The listing builds one solid part. Answer for the finished solid, in the listing's coordinates (mm). A direction names the side the tool comes from. Coordinates: 2 decimals unless noted, no trailing zeros. Write each loop counter-clockwise with the first axis right and the second up, starting at its lowest first coordinate (ties: lowest second). Pieces come first, ordered by that corner, then holes.
from build123d import *

# Parameters (mm, degrees)
F0_R     = 4
F0_R_2   = 3
F1_DEPTH = 2.5
F2_W     = 12
F2_H     = 2.5
F2_W_2   = 8
F3_DEPTH = 65.001


with BuildPart() as f1:
    # F0 (on Top) → F1 (new body, symmetric)
    with BuildSketch(Plane.XY):
        with BuildLine():
            ThreePointArc((45, -8), (53, 0), (45, 8))
            Line((45, 8), (15.268102, 8))
            ThreePointArc((15.268102, 8), (10.841623, 9.949533), (9.291666, 14.531239))
            Line((9.291666, 14.531239), (12, 45))
            ThreePointArc((12, 45), (0, 57), (-12, 45))
            Line((-12, 45), (-8, 0))
            ThreePointArc((-8, 0), (-5.656854, -5.656854), (0, -8))
            Line((0, -8), (45, -8))
        make_face()
        Circle(F0_R, mode=Mode.SUBTRACT)
        with Locations((45, 0)):
            Circle(F0_R_2, mode=Mode.SUBTRACT)
        with Locations((0, 45)):
            Circle(F0_R, mode=Mode.SUBTRACT)
    extrude(amount=F1_DEPTH, both=True)

    # F2 (on face) → F3 (cut, through all)
    with BuildSketch(Plane.XZ.offset(8)):
        with Locations((-6, 1.25)):
            Rectangle(F2_W, F2_H)
        with BuildLine():
            Line((0, 2.5), (0, 0))
            Line((0, 0), (17.572512, 0))
            ThreePointArc((17.572512, 0), (20.114295, 0.317372), (22.5, 1.25))
            ThreePointArc((22.5, 1.25), (24.885705, 2.182628), (27.427488, 2.5))
            Line((27.427488, 2.5), (0, 2.5))
        make_face()
        with BuildLine():
            ThreePointArc((22.5, -1.51663), (20.084839, -2.251757), (17.572512, -2.5))
            Line((17.572512, -2.5), (22.5, -2.5))
            Line((22.5, -2.5), (22.5, -1.51663))
        make_face()
        with BuildLine():
            Line((22.5, -1.51663), (22.5, -2.5))
            Line((22.5, -2.5), (45, -2.5))
            Line((45, -2.5), (45, 0))
            Line((45, 0), (27.427488, 0))
            ThreePointArc((27.427488, 0), (25.500431, -0.240616), (23.691705, -0.94769))
            ThreePointArc((23.691705, -0.94769), (23.103173, -1.247494), (22.5, -1.51663))
        make_face()
        with Locations((49, -1.25)):
            Rectangle(F2_W_2, F2_H)
    extrude(amount=-F3_DEPTH, mode=Mode.SUBTRACT)


solid = f1.part
Q1. The part is cut by section A-A, the plane y = 2. Write down the section's boundary in (x, z).
Answers below:
outline: (-8.18, -2.5) - (-3.46, -2.5) - (-3.46, 0) - (-8.18, 0) - close; (3.46, -2.5) - (17.57, -2.5) arc R12.84 ccw to (22.5, -1.52) arc R12.84 ccw to (23.69, -0.95) arc R7.84 cw to (27.43, 0) - (42.76, 0) - (42.76, 2.5) - (27.43, 2.5) arc R10.34 ccw to (22.5, 1.25) arc R10.34 cw to (17.57, 0) - (3.46, 0) - close; (47.24, 0) - (52.75, 0) - (52.75, 2.5) - (47.24, 2.5) - close
Q2. The part is cut by section D-D, the plane x = 11. Write down the section's boundary in (y, z), then the cut area to 3 significant figures.
Answers below:
outline: (-8, -2.5) - (9.78, -2.5) - (9.78, 0) - (-8, 0) - close; (33.75, -2.5) - (49.8, -2.5) - (49.8, 0) - (33.75, 0) - close
area: 84.6 mm2
Q3. Find the intervals of material crossed by probe 1 along Y at (x, z) = (-1, -1.45); probe 2 along Y at (x, z) = (45, 1.75); probe 3 along Y at (x, z) = (33, 2.35), in increasing order.
Answers below:
probe 1: y = -7.94 to -3.87, 3.87 to 41.13, 48.87 to 56.96
probe 2: y = -8 to -3, 3 to 8
probe 3: y = -8 to 8
Q4. Determine the mould class of faces 4 (the face through (3, 24, 0)), 5 (the face through (10.627, 29.552, -1.232)), 6 (the face through (22, -8, 0)) for opening direction Y: released by +Y, released by -Y, zero draft, split by the parting line, or undercut.
Answers below:
face 4: zero draft
face 5: undercut
face 6: released by -Y
Q5. Which of the six approach directions +Z, -Z, +X, -X, +Y, -Y give full straight-line access (tool end or side, diameter ignored) to faces 1 (the face through (10.89, 9.9, -1.23)), 2 (the face through (40, 0, 0)), 3 (the face through (30, 8, 1))?
Answers below:
face 1: +Z, -Z, +X
face 2: -Z, +X, +Y, -Y
face 3: +Z, -Z, +X, +Y
Q6. The part is cut by section B-B, the plane x = 43. Write down the section's boundary in (y, z).
Answers below:
outline: (-8, 0) - (-2.24, 0) - (-2.24, 2.5) - (-8, 2.5) - close; (2.24, 0) - (8, 0) - (8, 2.5) - (2.24, 2.5) - close
Q7. The part is cut by section C-C, the plane x = 3. Write down the section's boundary in (y, z), then the cut area to 3 significant figures.
Answers below:
outline: (-8, -2.5) - (-2.65, -2.5) - (-2.65, 0) - (-8, 0) - close; (2.65, -2.5) - (42.35, -2.5) - (42.35, 0) - (2.65, 0) - close; (47.65, -2.5) - (56.62, -2.5) - (56.62, 0) - (47.65, 0) - close
area: 135 mm2
Q8. Given pin 1 (1 mm diameter, centred on x = -5.5, y = 41.5, fed in from +Z); pin 2 (5.5 mm diameter, centred on x = 45, y = 0, fed in from -Z); pin 3 (13 mm diameter, centred on x = 38.5, y = -3.5, fed in from -Z); pin 4 (1 mm diameter, centred on y = 3.5, z = -1.5, fed in from -X), each flat-ended and moving along its own axis, determine where each tip first touches the part or whether it passes through.
Answers below:
pin 1: stops at z = 0
pin 2: passes through
pin 3: stops at z = 0
pin 4: stops at x = -8.36
